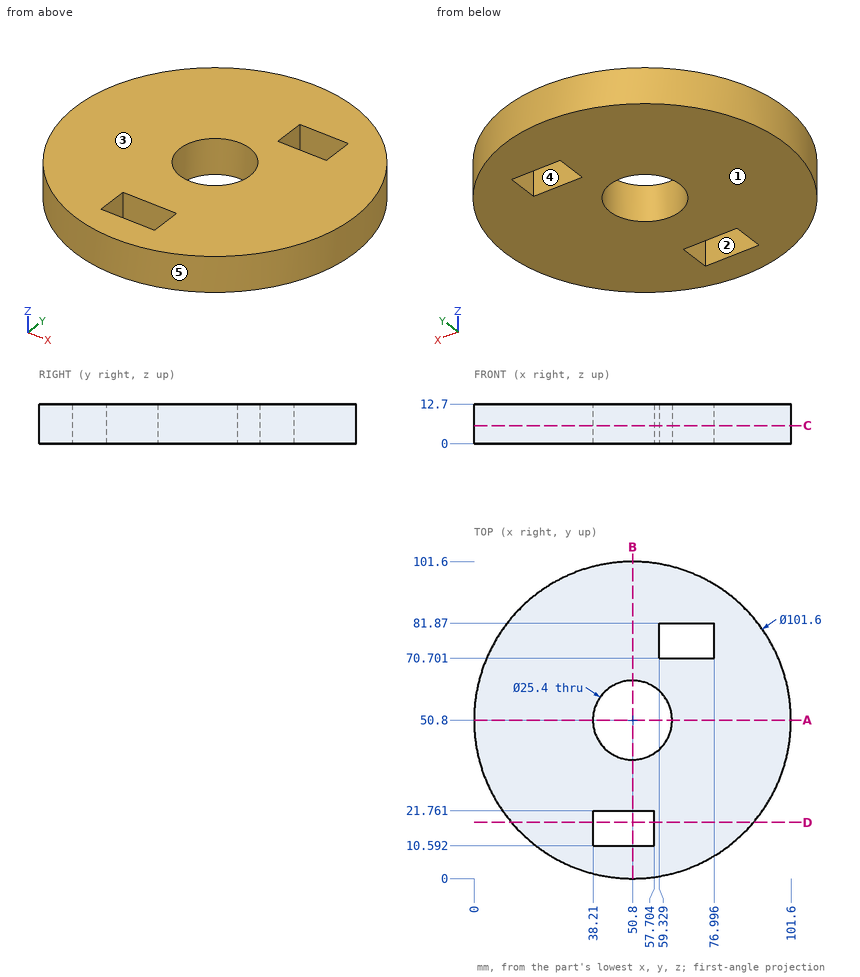
Input: dimensioned drawing with shaded views. Units: mm. Origin: part minimum x, y, z. A direction names the side the tool comes from. Round coordinates to 2 decimals unless told otherwise and drop trailing zeros. Order: outer loops, then holes, each group sorted by start corner. A loop starts at its lowest first (then second) coordinate and runs counter-clockwise, first axis right, second up. Notation, with made-up numbers: (1.5, -11) - (9.5, -11) arc R30 cw to (9.5, 12) - close; hole circle Ø11 at (-10.5, -20). An arc over 180 degrees is marked (long way). Use CSV: the item, a comma, the result in double quotes. Start each with the question number.
Q1. Material intervals for line 1 along Y through (x, z) = (50.8, 9.25); line 2 along X through (y, z) = (48, 12); line 3 along X through (y, z) = (56, 12), sorted ascending. Write a range as from..to.
Q2. Mould query, pull axis Y, two halves, no side actions, for the marked faces 3, 4 and 5. Classes: +Y half, -Y half, draft (parallel to the pull), parting line (faces both ways), or undercut.
Q3. Section query B-B (x = 50.8). Return loops of the section in (y, z), and give its area (3 significant figures).
Q4. First-contact query: pin 1 (4 mm diameter, centred on x = 65.5, z = 5.5, fed in from -Y); pin 2 (1.5 mm diameter, centred on x = 84.5, y = 14, fed in from -Z); pin 3 (4 mm diameter, centred on x = 44, z = 7, fed in from -Y); pin 4 (5.5 mm diameter, centred on y = 15.5, z = 8, fed in from +X). Flat tips, straight axial feed; report the tip coordinate or a pass-through.
Q5. Section query D-D (y = 18). Return loops of the section in (x, z) (1 decimal).
Q6. Section query C-C (z = 5.75). Return loops of the section in (x, y) (1 decimal), and give its area (3 significant figures).
Q7. Section query A-A (y = 50.8). Return loops of the section in (x, z).
Q8. Access query for the marked faces 1 and 2. Directions: +Z, -Z, +X, -X, +Y, -Y. A direction counts if a zero-diameter tool reaches every point of the face in a straight line with its end or side. Return the directions, or none.
Result set:
1,line 1,"y = 0..10.59, 21.76..38.1, 63.5..101.6"
1,line 2,"x = 0.08..38.41, 63.19..101.52"
1,line 3,"x = 0.27..39.21, 62.39..101.33"
2,face 3,"draft"
2,face 4,"undercut"
2,face 5,"parting line"
3,outline,"(0, 0) - (10.59, 0) - (10.59, 12.7) - (0, 12.7) - close; (21.76, 0) - (38.1, 0) - (38.1, 12.7) - (21.76, 12.7) - close; (63.5, 0) - (101.6, 0) - (101.6, 12.7) - (63.5, 12.7) - close"
3,area,"826 mm2"
4,pin 1,"stops at y = 1.61"
4,pin 2,"stops at z = 0"
4,pin 3,"stops at y = 0.23"
4,pin 4,"stops at x = 89.8"
5,outline,"(12, 0) - (38.2, 0) - (38.2, 12.7) - (12, 12.7) - close; (57.7, 0) - (89.6, 0) - (89.6, 12.7) - (57.7, 12.7) - close"
6,outline,"circle Ø101.6 at (50.8, 50.8); hole circle Ø25.4 at (50.8, 50.8); hole (38.2, 10.6) - (57.7, 10.6) - (57.7, 21.8) - (38.2, 21.8) - close; hole (59.3, 70.7) - (77, 70.7) - (77, 81.9) - (59.3, 81.9) - close"
6,area,"7,190 mm2"
7,outline,"(0, 0) - (38.1, 0) - (38.1, 12.7) - (0, 12.7) - close; (63.5, 0) - (101.6, 0) - (101.6, 12.7) - (63.5, 12.7) - close"
8,face 1,"-Z, +X, -X, +Y, -Y"
8,face 2,"+Z, -Z"
